CAD build for the part. Positions are in the model's coordinates, mm. Face numbers are marked on the shaded views. Coordinates: 2 decimals unless noted, no trailing zeros. Loops run counter-clockwise (first coordinate to the right, second up) from the corner with the lowest first, then second, coordinate; pieces in that order, holes last. Notation, with made-up numbers: (2, 2) -> (57, 2) arc R20 cw to (57, 24) -> close; hole circle Ø2 at (5, 9.25). An arc over 180 degrees is marked (long way). Write each question's results on one line, items separated by ' | '.
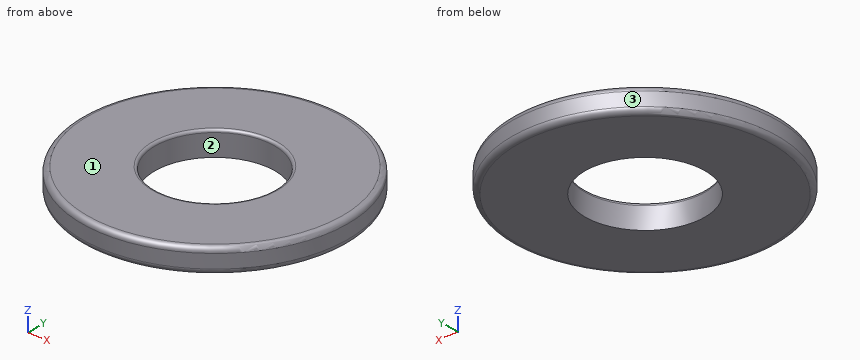
```python
from build123d import *

# Parameters (mm, degrees)
BOSS_EXTRUDE1_DEPTH      = 0.275
BOSS_EXTRUDE1_DEPTH_BACK = 0.275
SKETCH3_R                = 3
SKETCH3_R_2              = 1.35
FILLET1_R                = 0.12
FILLET2_R                = 0.06


with BuildPart() as part:
    # Sketch3 → Boss-Extrude1 (new, two sides: drawn at the far end of the back side and taken through both)
    with BuildSketch(Plane.XY.offset(-BOSS_EXTRUDE1_DEPTH_BACK)):
        Circle(SKETCH3_R)
        Circle(SKETCH3_R_2, mode=Mode.SUBTRACT)
    extrude(amount=BOSS_EXTRUDE1_DEPTH + BOSS_EXTRUDE1_DEPTH_BACK)

    # Fillet1
    fillet1_edges = [part.edges().sort_by_distance(p)[0] for p in [
        (-3, 0, -0.275),
        (-3, 0, 0.275),
    ]]
    fillet(fillet1_edges, radius=FILLET1_R)

    # Fillet2
    fillet2_edges = [part.edges().sort_by_distance(p)[0] for p in [
        (-1.35, 0, 0.275),
    ]]
    fillet(fillet2_edges, radius=FILLET2_R)


solid = part.part
```
Q1. Wall check: L1, parallel to Y at x = 0, z = 0.1; L2, parallel to Y at x = 1, z = 0.05; L3, parallel to X at y = -0.75, z = -0.2. Give the ranges that are in metal, low to high. Write a range as from..to.
Results are:
L1: -3..-1.35, 1.35..3 | L2: -2.83..-0.91, 0.91..2.83 | L3: -2.9..-1.12, 1.12..2.9
Q2. Pull direction Y, two halves, no side cores. Call the marked faces 1, 2 and 3: +Y half, -Y half, draft (parallel to the pull), parting line (faces both ways), or undercut.
Results are:
face 1: draft | face 2: undercut | face 3: parting line
Q3. Cut at A-A on x = 0. Write the cut outline in (y, z) (3 decimals), and give its area (3 significant figures).
Results are:
outline: (-3, -0.155) arc R0.12 ccw to (-2.88, -0.275) -> (-1.35, -0.275) -> (-1.35, 0.215) arc R0.06 ccw to (-1.41, 0.275) -> (-2.88, 0.275) arc R0.12 ccw to (-3, 0.155) -> close; (1.35, -0.275) -> (2.88, -0.275) arc R0.12 ccw to (3, -0.155) -> (3, 0.155) arc R0.12 ccw to (2.88, 0.275) -> (1.41, 0.275) arc R0.06 ccw to (1.35, 0.215) -> close | area: 1.80 mm^2
Q4. Cut at C-C on z = 0. Write the cut outline in (x, y), and give its area (3 significant figures).
Results are:
outline: circle Ø6 at (0, 0); hole circle Ø2.7 at (0, 0) | area: 22.5 mm^2
